Work out the finished part from the listing and answer in its coordinate system (mm). A direction names the side the tool comes from. Coordinates: 2 decimals unless noted, no trailing zeros. Order: outer loops, then holes, each group sorted by start corner. A loop starts at its lowest first (then second) coordinate and runs counter-clockwise, first axis right, second up.
```python
from build123d import *


with BuildPart() as part:
    # Sketch2 → Revolve1 (revolve)
    with BuildSketch(Plane.XY):
        with BuildLine():
            Line((-152.4, 0), (0, 0))
            Line((0, 0), (0, -5.588))
            Line((0, -5.588), (-6.35, -5.588))
            Line((-6.35, -5.588), (-6.35, -7.9502))
            Line((-6.35, -7.9502), (-19.05, -7.9502))
            Line((-19.05, -7.9502), (-19.05, -5.842))
            Line((-19.05, -5.842), (-22.86, -5.842))
            Line((-22.86, -5.842), (-22.86, -7.9502))
            Line((-22.86, -7.9502), (-65.849197896, -11.7094))
            ThreePointArc((-65.849197896, -11.7094), (-66.889567891, -12.222411886), (-67.31, -13.303516767))
            Line((-67.31, -13.303516767), (-67.31, -15.875))
            Line((-67.31, -15.875), (-92.71, -15.875))
            Line((-92.71, -15.875), (-92.71, -17.4752))
            Line((-92.71, -17.4752), (-95.885, -17.4752))
            Line((-95.885, -17.4752), (-95.885, -19.05))
            ThreePointArc((-95.885, -19.05), (-96.81493597, -21.29506403), (-99.06, -22.225))
            Line((-99.06, -22.225), (-121.285, -22.225))
            Line((-121.285, -22.225), (-121.285, -25.4))
            Line((-121.285, -25.4), (-152.4, -25.4))
            Line((-152.4, -25.4), (-152.4, 0))
        make_face()
    revolve(axis=Axis((88.99, 0, 0), (-1, 0, 0)))


solid = part.part
```
1. For faces 1 (the flat face through (-19.05, 0, 6)), 2 (the cylindrical face through (-3.219, 4.434, -3.4)), 3 (the flat face through (-152.4, 0, 0)), determine the directions among +Z, -Z, +X, -X, +Y, -Y from which every point of the face is accessible in a straight line to the end or side of a thin tool.
2. Flat-ended cylindrical pins translate along their axes: pin 1 (5 mm diameter, centred on y = -0.5, z = 1.5, fed in from +X); pin 2 (1 mm diameter, centred on y = 19, z = -14, fed in from +X) (3 decimals); pin 3 (4 mm diameter, centred on x = -43.5, y = 4.5, fed in from +Z); pin 4 (6 mm diameter, centred on x = -79, y = -3.5, fed in from +Z). Find the tip coordinate at first contact, or state that the pin passes through.
3. The part is cut by section A-A (x = -57.5). Determine the outline of the cut face in (y, z).
4. Consider probe 1 along X at (y, z) = (-2, 22.5) (3 decimals); probe 2 along X at (y, z) = (9, 13.5); probe 3 along Y at (x, z) = (-99.5, 1). Determine where each line is inside the solid, lowest interval first.
5. The part is cut by section B-B (x = -101). Determine the outline of the cut face in (y, z) (3 decimals).
Worked out:
1. face 1: none
1. face 2: +X
1. face 3: +Z, -Z, -X, +Y, -Y
2. pin 1: stops at x = 0
2. pin 2: stops at x = -121.285
2. pin 3: stops at z = 9.46
2. pin 4: stops at z = 15.87
3. outline: circle Ø21.96 at (0, 0)
4. probe 1: x = -152.4 to -121.285
4. probe 2: x = -152.4 to -92.71
4. probe 3: y = -22.2 to 22.2
5. outline: circle Ø44.45 at (0, 0)
